Print and shaded views of the part. All mm, measured from the part's lowest x, y and z. A direction names the side the tool comes from. Coordinates: 2 decimals unless noted, no trailing zeros. Order: outer loops, then holes, each group sorted by start corner. A loop starts at its lowest first (then second) coordinate and runs counter-clockwise, first axis right, second up. Notation, with made-up numbers: (-1, 10.25) -> (45, 10.25) arc R25 ccw to (45, 35.25) -> close; hole circle Ø2 at (64, 6.25). An arc over 180 degrees is marked (long way). Use one line per item in the form item = value. Start each with the question number.
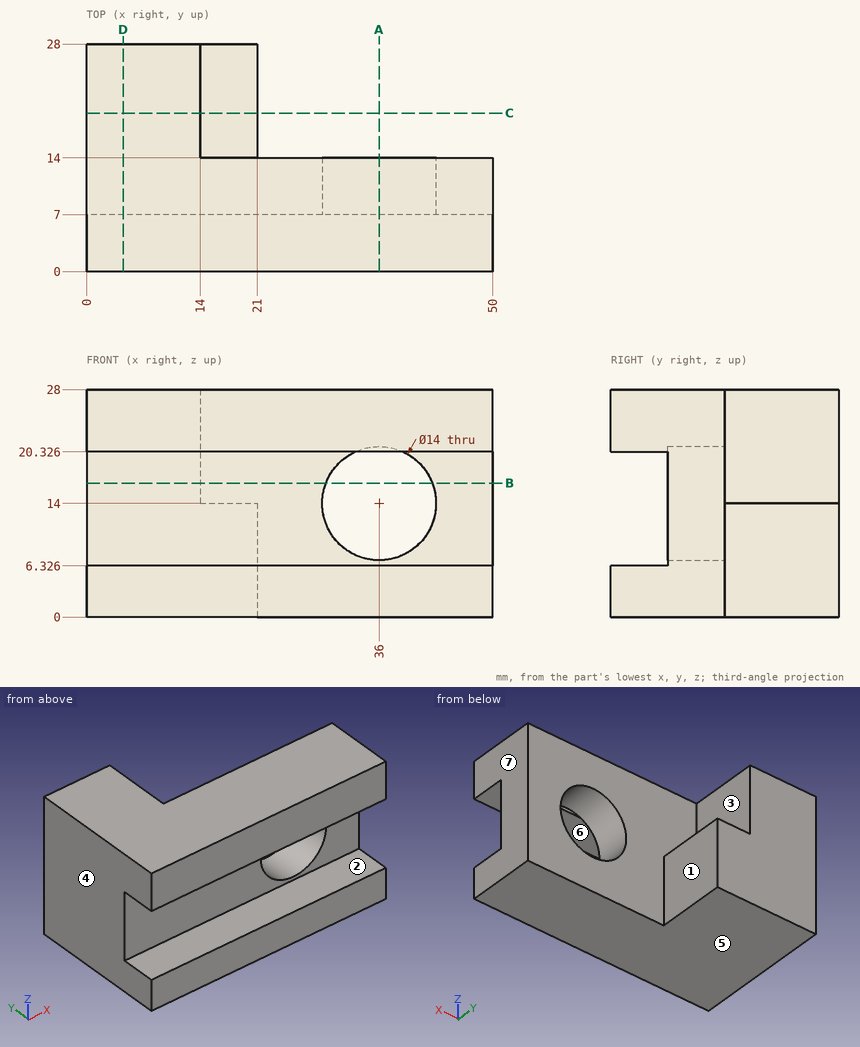
1) 3-axis set-ups, long thin cutter, end or side, ignore diameter. For the marked faces 1, 2, 3 and 4: which of +Z, -Z, +X, -X, +Y, -Y reach the whole face in a straight line?
2) Cut at D-D on x = 4.5. Give the cut face in (y, z), then the cut area to 3 significant figures.
3) Cut at B-B on z = 16.5. Give the cut face in (x, y).
4) Drop flat-ended pins along their axis: P1, Ø2, axis at x = 16.5, y = 23.5, coming from the +Z side; P2, Ø12.5, axis at x = 36, z = 14, coming from the -Y side; P3, Ø6, axis at x = 38, z = 10.5, coming from the +Y side; P4, Ø11, axis at y = 20.5, z = 9, coming from the +X side. Give the stop position or say it passes through.
5) Cut at A-A on x = 36. Give the cut face in (y, z).
6) Two-plate mould, pull along Z, no slides. Class the marked faces 5, 6 and 7: released by +Z, released by -Z, zero draft, split by the parting line, or undercut.
7) Probe L1, parallel to X at y = 10.75, z = 14; L2, parallel to Z at x = 36, y = 10.5; L3, parallel to X at y = 14.75, z = 20. List the from-to ranges inside material, lowest first.
8) Cut at C-C on y = 19.5. Give the cut face in (x, z), then the cut area to 3 significant figures.
Values follow:
q1.face_1 = +Z, -Z, +X, +Y
q1.face_2 = +X, -X, -Y
q1.face_3 = +Z, +X, +Y
q1.face_4 = +Z, -Z, -X, +Y, -Y
q2.outline = (0, 0) -> (28, 0) -> (28, 28) -> (0, 28) -> (0, 20.33) -> (7, 20.33) -> (7, 6.33) -> (0, 6.33) -> close
q2.area = 686 mm^2
q3.outline = (0, 7) -> (29.46, 7) -> (29.46, 14) -> (14, 14) -> (14, 28) -> (0, 28) -> close; (42.54, 7) -> (50, 7) -> (50, 14) -> (42.54, 14) -> close
q4.P1 = 14
q4.P2 = through
q4.P3 = 14
q4.P4 = 21
q5.outline = (0, 0) -> (14, 0) -> (14, 7) -> (7, 7) -> (7, 6.33) -> (0, 6.33) -> close; (0, 20.33) -> (7, 20.33) -> (7, 21) -> (14, 21) -> (14, 28) -> (0, 28) -> close
q6.face_5 = released by -Z
q6.face_6 = undercut
q6.face_7 = zero draft
q7.L1 = 0 to 29, 43 to 50
q7.L2 = 0 to 7, 21 to 28
q7.L3 = 0 to 14
q8.outline = (0, 0) -> (21, 0) -> (21, 14) -> (14, 14) -> (14, 28) -> (0, 28) -> close
q8.area = 490 mm^2
